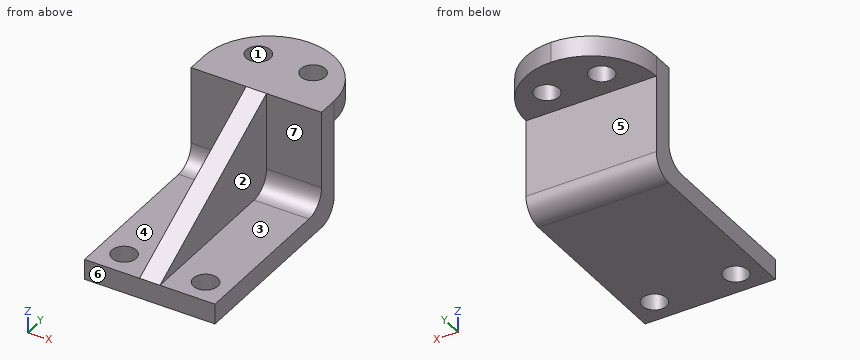
from build123d import *

# Parameters (mm, degrees)
F1_DEPTH = 5
F2_DEPTH = 32
F4_R     = 6
F5_DEPTH = 58.001


with BuildPart() as f1:
    # F0 (on Right) → F1 (new body, symmetric)
    with BuildSketch(Plane.YZ):
        with BuildLine():
            Line((85, 48), (0, 0))
            Line((0, 0), (75, 0))
            ThreePointArc((75, 0), (82.0710678119, 2.9289321881), (85, 10))
            Line((85, 10), (85, 48))
        make_face()
        with BuildLine():
            Line((75, 0), (0, 0))
            Line((0, 0), (0, -10))
            Line((0, -10), (85, -10))
            ThreePointArc((85, -10), (92.0710678119, -7.0710678119), (95, 0))
            Line((95, 0), (95, 38))
            Line((95, 38), (127, 38))
            Line((127, 38), (127, 48))
            Line((127, 48), (85, 48))
            Line((85, 48), (85, 10))
            ThreePointArc((85, 10), (82.0710678119, 2.9289321881), (75, 0))
        make_face()
    extrude(amount=F1_DEPTH, both=True)

    # F0 (on Right) → F2 (join, symmetric)
    with BuildSketch(Plane.YZ):
        with BuildLine():
            Line((75, 0), (0, 0))
            Line((0, 0), (0, -10))
            Line((0, -10), (85, -10))
            ThreePointArc((85, -10), (92.0710678119, -7.0710678119), (95, 0))
            Line((95, 0), (95, 38))
            Line((95, 38), (127, 38))
            Line((127, 38), (127, 48))
            Line((127, 48), (85, 48))
            Line((85, 48), (85, 10))
            ThreePointArc((85, 10), (82.0710678119, 2.9289321881), (75, 0))
        make_face()
    extrude(amount=F2_DEPTH, both=True)

    # F4 (on face) → F5 (cut, through all)
    with BuildSketch(Plane.XY.offset(48)):
        with BuildLine():
            ThreePointArc((-32, 95), (-22.6274171136, 117.6274168823), (-3.272e-07, 127))
            Line((-3.272e-07, 127), (-32, 127))
            Line((-32, 127), (-32, 95))
        make_face()
        with BuildLine():
            ThreePointArc((-3.272e-07, 127), (22.6274168823, 117.6274171136), (32, 95))
            Line((32, 95), (32, 127))
            Line((32, 127), (-3.272e-07, 127))
        make_face()
        with Locations((13.4350288425, 108.4350288425)):
            Circle(F4_R)
        with Locations((-13.4350288425, 108.4350288425)):
            Circle(F4_R)
        with Locations((-20, 12)):
            Circle(F4_R)
        with Locations((20, 12)):
            Circle(F4_R)
    extrude(amount=-F5_DEPTH, mode=Mode.SUBTRACT)


solid = f1.part
Model file for the job. Use its own axes, mm. Face numbers are marked on the shaded views. A direction names the side the tool comes from. Coordinates: 2 decimals unless noted, no trailing zeros. Write each loop counter-clockwise with the first axis right and the second up, starting at its lowest first coordinate (ties: lowest second). Pieces come first, ordered by that corner, then holes. Notation, with made-up numbers: (-5.5, 16) -> (14.5, 16) arc R28 cw to (14.5, 53) -> close; hole circle Ø3 at (44.25, -22.5). An arc over 180 degrees is marked (long way). One line per item, written item: value. Start each with the question number.
1) Slice it at C-C on y = 12. Write the cut outline in (x, z).
2) Which spindle directions (+Z, -Z, +X, -X, +Y, -Y) get a long thin tool onto all of the face, cutting with end or side? Do the marked faces 4, 5, 6 and 7. Say none if no direction does.
3) Pull direction X, two halves, no side cores. Call the marked faces 1, 2 and 3: +X half, -X half, draft (parallel to the pull), parting line (faces both ways), or undercut.
4) Slice it at D-D on x = -12.5. Write the cut outline in (y, z), then the cut area to 3 significant figures.
5) Probe probe 1 along Y at (x, z) = (29, 32); probe 2 along Z at (x, y) = (17, 18); probe 3 along Y at (x, z) = (20, -5.75). List the from-to ranges inside material, lowest first.
6) Slice it at A-A on x = 17. Write the cut outline in (y, z), then the cut area to 3 significant figures.
7) Flat gauge pins, fed straight in: pin 1 Ø24 at (y, z) = (48.5, 31) entering from +X; pin 2 Ø8 at (x, y) = (22, 52.5) entering from +Z; pin 3 Ø1 at (y, z) = (78, 36.5) entering from -X. Where does each tip first touch, or does it go through?
8) Slice it at B-B on z = 41.5. Write the cut outline in (x, y).
Answers follow:
1. outline: (-32, -10) -> (-26, -10) -> (-26, 0) -> (-32, 0) -> close; (-14, -10) -> (14, -10) -> (14, 0) -> (5, 0) -> (5, 6.78) -> (-5, 6.78) -> (-5, 0) -> (-14, 0) -> close; (26, -10) -> (32, -10) -> (32, 0) -> (26, 0) -> close
2. face 4: +Z, -X, -Y
2. face 5: -Z, +X, -X, +Y
2. face 6: +Z, -Z, +X, -X, -Y
2. face 7: +Z, +X, -Y
3. face 1: undercut
3. face 2: +X half
3. face 3: draft
4. outline: (0, -10) -> (85, -10) arc R10 ccw to (95, 0) -> (95, 38) -> (102.51, 38) -> (102.51, 48) -> (85, 48) -> (85, 10) arc R10 cw to (75, 0) -> (0, 0) -> close; (114.36, 38) -> (124.46, 38) -> (124.46, 48) -> (114.36, 48) -> close
4. area: 1,610 mm2
5. probe 1: 85 to 95
5. probe 2: -10 to 0
5. probe 3: 0 to 6, 18 to 93.18
6. outline: (0, -10) -> (6.8, -10) -> (6.8, 0) -> (0, 0) -> close; (17.2, -10) -> (85, -10) arc R10 ccw to (95, 0) -> (95, 38) -> (103.61, 38) -> (103.61, 48) -> (85, 48) -> (85, 10) arc R10 cw to (75, 0) -> (17.2, 0) -> close; (113.26, 38) -> (122.11, 38) -> (122.11, 48) -> (113.26, 48) -> close
6. area: 1,500 mm2
7. pin 1: x = 5
7. pin 2: z = 0
7. pin 3: x = -5
8. outline: (-32, 85) -> (-5, 85) -> (-5, 73.49) -> (5, 73.49) -> (5, 85) -> (32, 85) -> (32, 95) arc R32 ccw to (-32, 95) -> close; hole circle Ø12 at (-13.44, 108.44); hole circle Ø12 at (13.44, 108.44)
